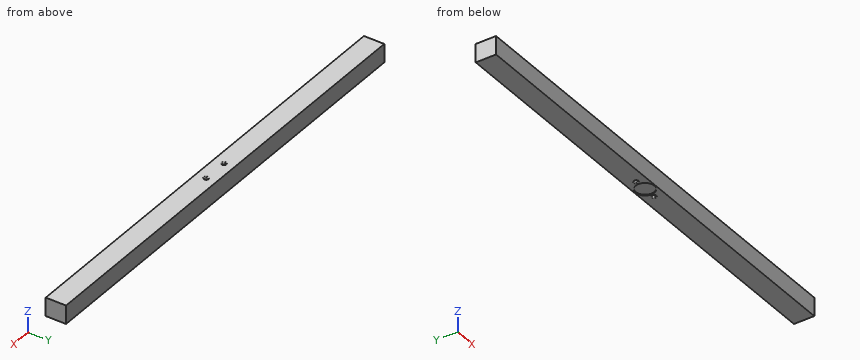
Solid Edge part; units mm, degrees
sketch "Sketch1" plane through (0, 0, 0) normal (1, 0, 0) x (0, 1, 0)
  line L0 (-126.3361, -70.1543) -> (-16.3361, -70.1543)
  line L1 (-16.3361, -70.1543) -> (-16.3361, 29.8457)
  line L2 (-16.3361, 29.8457) -> (-126.3361, 29.8457)
  line L3 (-126.3361, 29.8457) -> (-126.3361, -70.1543)
extrude "Protrusion1" add sketch "Sketch1" against normal blind 2500
sketch "Sketch2" plane through (-1250, -71.3361, -70.1543) normal (0, 0, -1) x (1, 0, 0)
  circle A0 centre (0, 0) radius 50
extrude "ExtrudedCutout_2" cut sketch "Sketch2" against normal blind 5
sketch "Sketch3" plane through (-1250, -71.3361, 29.8457) normal (0, 0, 1) x (1, 0, 0)
  circle A0 centre (-70, 0) radius 10
  circle A1 centre (70, 0) radius 10
extrude "Cutout1" cut sketch "Sketch3" against normal through all
fillet "Round_1" radius 5 4 edges at (-1330, -71.3361, 29.8457) (-1310, -71.3361, -70.1543) (-1190, -71.3361, 29.8457) (-1170, -71.3361, -70.1543)
Check sheet for the modelled part. Datum: model origin and axes. Units: mm. Round coordinates to 2 decimals unless told otherwise and drop trailing zeros. Write each loop counter-clockwise with the first axis right and the second up, starting at its lowest first coordinate (ties: lowest second). Pieces come first, ordered by that corner, then holes. Notation, with made-up numbers: M 22,-5.75 L 78,-5.75 A16 ccw 78,8.25 Z; hole C -30,84.5 d9. An arc over 180 degrees is marked long. Write item = value, one per line. Start each with the question number.
1. Scan lines: line 1 (X direction, y = -72, z = 15); line 2 (Y direction, x = -1250, z = -67.7); line 3 (X direction, y = -64, z = 5.5). Record each from-to range of solid material in increasing order. Write a range as [from, to].
2. Section check A-A, the plane x = -1250. Record the cut outline in (y, z).
3. Gauge pin test, flat end, axial feed: pin 1 (23 mm diameter, centred on x = -1180, y = -71.34, fed in from -Z). Record the tip position at first contact, or that the pin passes through.
Results found:
q1.line_1 = [-2500, -1329.98], [-1310.02, -1189.98], [-1170.02, 0]
q1.line_2 = [-126.34, -121.34], [-21.34, -16.34]
q1.line_3 = [-2500, -1326.8], [-1313.2, -1186.8], [-1173.2, 0]
q2.outline = M -126.34,-70.15 L -121.34,-70.15 L -121.34,-65.15 L -21.34,-65.15 L -21.34,-70.15 L -16.34,-70.15 L -16.34,29.85 L -126.34,29.85 Z
q3.pin_1 = -68.73
